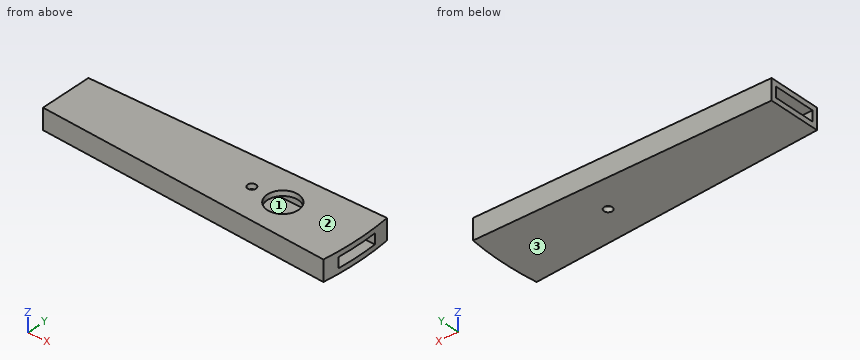
from build123d import *

# Parameters (mm, degrees)
F0_R     = 7.5
F1_DEPTH = 10
F2_W     = 20
F2_H     = 5
F3_DEPTH = 200
F4_R     = 7.5
F5_DEPTH = 2.5
F6_R     = 2
F7_DEPTH = 10


with BuildPart() as f1:
    # F0 (on Top) → F1 (new body)
    with BuildSketch(Plane.XY):
        with BuildLine():
            Line((70, 17.5), (-70, 12.5))
            Line((-70, 12.5), (-70, -12.5))
            Line((-70, -12.5), (70, -17.5))
            ThreePointArc((70, -17.5), (71.089511, 0), (70, 17.5))
        make_face()
        with Locations((35, 0)):
            Circle(F0_R, mode=Mode.SUBTRACT)
        with Locations((35, 0)):
            Circle(F0_R)
    extrude(amount=F1_DEPTH)

    # F2 (on face) → F3 (cut)
    with BuildSketch(Plane(origin=(-70, 0, 0), x_dir=(0, -1, 0), z_dir=(-1, 0, 0))):
        with Locations((0, 5)):
            Rectangle(F2_W, F2_H)
    extrude(amount=-F3_DEPTH, mode=Mode.SUBTRACT)

    # F4 (on face) → F5 (cut)
    with BuildSketch(Plane.XY.offset(10)):
        with Locations((35, 0)):
            Circle(F4_R)
    extrude(amount=-F5_DEPTH, mode=Mode.SUBTRACT)

    # F6 (on face) → F7 (cut)
    with BuildSketch(Plane.XY.offset(10)):
        with Locations((20, 0)):
            Circle(F6_R)
    extrude(amount=-F7_DEPTH, mode=Mode.SUBTRACT)


solid = f1.part
The model under review builds one solid part; all positions refer to its coordinate system, in mm. Face numbers are marked on the shaded views. Round coordinates to 2 decimals unless told otherwise and drop trailing zeros. Loops run counter-clockwise (first coordinate to the right, second up) from the corner with the lowest first, then second, coordinate; pieces in that order, holes last. Notation, with made-up numbers: (13, 44) -> (47, 44) arc R24 cw to (47, 57) -> close; hole circle Ø11 at (-3, 52). An arc over 180 degrees is marked (long way). Answer as CSV lines item,"result".
1) Draft analysis for pull direction Z (two halves, no side actions). For the marked faces 1, 2 and 3, state which applies: pulls with the +Z half, pulls with the -Z half, needs draft (parallel to the pull), parting line crosses it, or undercut.
Geometry results:
face 1,"undercut"
face 2,"pulls with the +Z half"
face 3,"pulls with the -Z half"
2) To check wall thickness, follow line 1 along Z through (x, y) = (39.5, -7); line 2 along Y through (x, z) = (20, 8.8); line 3 along Z through (x, y) = (30, -5.5). State the ranges of each line that lie inside material, in increasing order. Write a range as from..to.
Geometry results:
line 1,"z = 0..2.5, 7.5..10"
line 2,"y = -15.71..-2, 2..15.71"
line 3,"z = 0..2.5"
3) Add section A-A on z = 6. Write out the cut boundary in (x, y).
Geometry results:
outline,"(-70, -12.5) -> (70, -17.5) arc R141.09 ccw to (70.73, -10) -> (-70, -10) -> close; (-70, 10) -> (70.73, 10) arc R141.09 ccw to (70, 17.5) -> (-70, 12.5) -> close"
4) Add section B-B on x = 35. Write out the cut boundary in (y, z).
Geometry results:
outline,"(-16.25, 0) -> (16.25, 0) -> (16.25, 10) -> (7.5, 10) -> (7.5, 7.5) -> (10, 7.5) -> (10, 2.5) -> (-10, 2.5) -> (-10, 7.5) -> (-7.5, 7.5) -> (-7.5, 10) -> (-16.25, 10) -> close"
5) Add section D-D on x = -46.5. Write out the cut boundary in (y, z), plus the area to 3 significant figures.
Geometry results:
outline,"(-13.34, 0) -> (13.34, 0) -> (13.34, 10) -> (-13.34, 10) -> close; hole (-10, 2.5) -> (10, 2.5) -> (10, 7.5) -> (-10, 7.5) -> close"
area,"167 mm²"
6) For P1, Ø1.5, axis at x = -24.5, z = 6, coming from the -Y side; P2, Ø1.5, axis at x = -28, z = 5, coming from the +Y side; P3, Ø4, axis at x = -14, z = 8, coming from the +Y side; P4, Ø1.5, axis at x = 38, y = -2.5, coming from the -Z side, all flat-tipped, find the tip position at first contact; note any pin that passes through.
Geometry results:
P1,"stops at y = -14.15"
P2,"stops at y = 14.03"
P3,"stops at y = 14.57"
P4,"stops at z = 0"
7) Add section C-C on y = 0. Write out the cut boundary in (x, z).
Geometry results:
outline,"(-70, 0) -> (18, 0) -> (18, 2.5) -> (-70, 2.5) -> close; (-70, 7.5) -> (18, 7.5) -> (18, 10) -> (-70, 10) -> close; (22, 0) -> (71.09, 0) -> (71.09, 2.5) -> (22, 2.5) -> close; (22, 7.5) -> (27.5, 7.5) -> (27.5, 10) -> (22, 10) -> close; (42.5, 7.5) -> (71.09, 7.5) -> (71.09, 10) -> (42.5, 10) -> close"
